CAD build for the part. Positions are in the model's coordinates, mm. A direction names the side the tool comes from. Round coordinates to 2 decimals unless told otherwise and drop trailing zeros. Write each loop counter-clockwise with the first axis right and the second up, starting at its lowest first coordinate (ties: lowest second). Pieces come first, ordered by that corner, then holes. Notation, with made-up numbers: (18, 19) -> (54, 19) arc R36 cw to (54, 55) -> close; hole circle Ø10 at (68, -20.75). An arc over 180 degrees is marked (long way). Answer in a Markdown table with one row per item. Add a question column.
```python
from build123d import *

# Parameters (mm, degrees)
F1_DEPTH = 39
F2_R     = 2.5
F3_DEPTH = 2.748386896
F4_R     = 12.0181970212
F5_DEPTH = 5.3
F6_R     = 10.1005312929
F7_DEPTH = 1
F8_R     = 8.272494484
F9_DEPTH = 1
F10_R    = 0.49999


# Not quite as in the source:
# - a fillet or chamfer is up to 0.001 mm smaller than in the source, because OpenCascade refuses the exact size


with BuildPart() as f1:
    # F0 (on Front) → F1 (new body, symmetric)
    with BuildSketch(Plane.XZ):
        Polygon((33.0240737289, -6.6249261405), (-2.9748248395, -6.6249261405), (-2.9748248395, -9.6249261405), (36.0251751605, -9.6249261405), (36.0251751605, 18.3750738595), (48.0240737289, 18.3750738595), (48.0240737289, 21.1234607555), (33.0240737289, 21.1234607555), align=None)
        Polygon((-2.9748248395, -9.6249261405), (-2.9748248395, -6.6249261405), (-38.9737234078, -6.6249261405), (-38.9737234078, 21.1234607555), (-53.9737234078, 21.1234607555), (-53.9737234078, 18.3750738595), (-41.9748248395, 18.3750738595), (-41.9748248395, -9.6249261405), align=None)
    extrude(amount=F1_DEPTH, both=True)

    # F2 (on face) → F3 (cut, through all)
    with BuildSketch(Plane.XY.offset(21.1234607555)):
        with Locations((42.0246244447, -24)):
            Circle(F2_R)
        with Locations((42.0246244447, 24)):
            Circle(F2_R)
        with Locations((-47.9742741236, 24)):
            Circle(F2_R)
        with Locations((-47.9742741236, -24)):
            Circle(F2_R)
    extrude(amount=-F3_DEPTH, mode=Mode.SUBTRACT)

    # F4 (on face) → F5 (join)
    with BuildSketch(Plane(origin=(0, 0, -9.6249261405), x_dir=(1, 0, 0), z_dir=(0, 0, -1))):
        with Locations((-2.7290005237, -0.3212007869)):
            Circle(F4_R)
    extrude(amount=-F5_DEPTH)

    # F6 (on face) → F7 (cut)
    with BuildSketch(Plane.XY.offset(-4.3249261405)):
        with Locations((-2.7290005237, 0.3212007869)):
            Circle(F6_R)
    extrude(amount=-F7_DEPTH, mode=Mode.SUBTRACT)

    # F8 (on face) → F9 (cut)
    with BuildSketch(Plane.XY.offset(-5.3249261405)):
        with Locations((-2.7290005237, 0.3212007869)):
            Circle(F8_R)
    extrude(amount=-F9_DEPTH, mode=Mode.SUBTRACT)

    # F10 (radius 0.5 in the source; OpenCascade refuses exactly that, so slightly less here)
    f10_edges = [f1.edges().sort_by_distance(p)[0] for p in [
        (-14.747198, 0.321201, -4.324926),
        (-12.829532, 0.321201, -4.324926),
        (-12.829532, 0.321201, -5.324926),
        (-11.001495, 0.321201, -5.324926),
        (-11.001495, 0.321201, -6.324926),
    ]]
    fillet(f10_edges, radius=F10_R)


solid = f1.part
```
Item 1: Two-plate mould, pull along Y, no slides. Class faces 6 (the flat face through (-4, -1, -9.625)), 7 (the cylindrical face through (-46.63, 26.11, 19.77)), 8 (the flat face through (-3, 0, -6.325)), 9 (the flat face through (1, -39, -7)): +Y half, -Y half, draft (parallel to the pull), parting line (faces both ways), or undercut.
Item 2: Tool access for faces 1 (the flat face through (2, 10, -4.325)), 2 (the cylindrical face through (-11.59, -7.8, -5.74)), 3 (the cylindrical face through (39.527, 24.11, 19.769)), 4 (the flat face through (-41.975, -1, 5)), 5 (the flat face through (36.025, -1, 4)): list every direction of +Z, -Z, +X, -X, +Y, -Y with a clear straight run to the whole face (end or side of a thin tool).
Item 3: Pin check, flat tips, straight feed: pin 1 (8.5 mm diameter, centred on y = 4, z = 1, fed in from -X); pin 2 (8.5 mm diameter, centred on y = -11.5, z = 8.5, fed in from +X); pin 3 (12.5 mm diameter, centred on x = 1, y = -1.5, fed in from +Z); pin 4 (12 mm diameter, centred on y = 28.5, z = 14.5, fed in from -X). Stop position of each tip, or through.
Item 4: Drill centre lines: probe 1 along X at (y, z) = (18.5, 1); probe 2 along Z at (x, y) = (-30.5, -32); probe 3 along Z at (x, y) = (39.5, -9.5). Where is each one in solid material? Low to high.
Item 5: Saw through at A-A on z = 3.5. Give the cut face in (x, y).
Item 6: Saw through at C-C on x = -29.5. Give the cut face in (y, z), then the cut area to 3 significant figures.
Item 7: Saw through at B-B on y = -24. Give the cut face in (x, z), then the cut area to 3 significant figures.
Recorded:
| question | item | result |
|---|---|---|
| 1 | face 6 | draft |
| 1 | face 7 | undercut |
| 1 | face 8 | undercut |
| 1 | face 9 | -Y half |
| 2 | face 1 | +Z, +Y, -Y |
| 2 | face 2 | +Z |
| 2 | face 3 | +Z, -Z |
| 2 | face 4 | -Z, -X, +Y, -Y |
| 2 | face 5 | -Z, +X, +Y, -Y |
| 3 | pin 1 | x = -41.97 |
| 3 | pin 2 | x = 36.03 |
| 3 | pin 3 | z = -4.37 |
| 3 | pin 4 | x = -53.97 |
| 4 | probe 1 | -41.97 to -38.97, 33.02 to 36.03 |
| 4 | probe 2 | -9.62 to -6.62 |
| 4 | probe 3 | 18.38 to 21.12 |
| 5 | outline | (-41.97, -39) -> (-38.97, -39) -> (-38.97, 39) -> (-41.97, 39) -> close; (33.02, -39) -> (36.03, -39) -> (36.03, 39) -> (33.02, 39) -> close |
| 6 | outline | (-39, -9.62) -> (39, -9.62) -> (39, -6.62) -> (-39, -6.62) -> close |
| 6 | area | 234 mm2 |
| 7 | outline | (-53.97, 18.38) -> (-50.47, 18.38) -> (-50.47, 21.12) -> (-53.97, 21.12) -> close; (-45.47, 18.38) -> (-41.97, 18.38) -> (-41.97, -9.62) -> (36.03, -9.62) -> (36.03, 18.38) -> (39.52, 18.38) -> (39.52, 21.12) -> (33.02, 21.12) -> (33.02, -6.62) -> (-38.97, -6.62) -> (-38.97, 21.12) -> (-45.47, 21.12) -> close; (44.52, 18.38) -> (48.02, 18.38) -> (48.02, 21.12) -> (44.52, 21.12) -> close |
| 7 | area | 439 mm2 |
